Input: part model. Units: mm. Frame: model coordinates. Face numbers are marked on the shaded views. A direction names the side the tool comes from. Round coordinates to 2 decimals unless told otherwise and drop trailing zeros. Loops run counter-clockwise (first coordinate to the right, second up) from the corner with the lowest first, then second, coordinate; pieces in that order, holes last. Notation, with made-up numbers: (13, 80.25) -> (48, 80.25) arc R30 cw to (48, 109.25) -> close; hole circle Ø2 at (11, 43). An arc over 180 degrees is marked (long way). Answer in a Markdown table with one row per item. Add a question column.
Q1. Section C-C, the plane x = 53.5. Output: boundary loops of the cut face in (y, z).
Q2. Section A-A, the plane y = 12.25. Output: boundary loops of the cut face in (x, z).
Q3. Section B-B, the plane x = 0. Output: boundary loops of the cut face in (y, z), and give its area (3 significant figures).
Q4. Reachability of the marked faces 1, 2 and 3 from +Z, -Z, +X, -X, +Y, -Y: full face, straight path, thin tool, end or side. Return the list, or none.
Q5. Pin query (flat end, axial travel): pin 1 (10 mm diameter, centred on x = 30.5, z = -108.5, fed in from -Y); pin 2 (3.5 mm diameter, centred on y = 9, z = -149, fed in from -X); pin 3 (13 mm diameter, centred on y = 15.5, z = -151, fed in from +X); pin 4 (9 mm diameter, centred on x = 0, y = 10, fed in from -Z). Return the tip coordinate at first contact, or that it passes through.
Q6. Section D-D, the plane z = -33.5. Output: boundary loops of the cut face in (x, y).
Q7. Ray query, L1, parallel to X at y = 9, z = -76.5; L2, parallel to X at y = 9.5, z = -77; L3, parallel to X at y = 12, z = -10. Return the intervals inside material, ascending. Write a range as from..to.
```python
from build123d import *

# Parameters (mm, degrees)
BOSS_EXTRUDE1_DEPTH = 2
SKETCH2_W           = 8
SKETCH2_H           = 12
BOSS_EXTRUDE2_DEPTH = 20
SKETCH6_W           = 4
SKETCH6_H           = 2.75
CUT_EXTRUDE3_DEPTH  = 20
SKETCH7_R           = 2
CUT_EXTRUDE4_DEPTH  = 10


with BuildPart() as part:
    # Sketch1 → Boss-Extrude1 (new body)
    with BuildSketch(Plane(origin=(0, 0, 0), x_dir=(1, 0, 0), z_dir=(0, 1, 0))):
        with BuildLine():
            Line((75.074639149, 80.253787975), (10.139177746, 145.189249379))
            ThreePointArc((10.139177746, 145.189249379), (-8.838834765, 161.338834765), (7.310750621, 142.360822254))
            Line((7.310750621, 142.360822254), (71.4177849, 78.253787975))
            Line((71.4177849, 78.253787975), (7.310750621, 14.146753697))
            ThreePointArc((7.310750621, 14.146753697), (-8.838834765, -4.831258814), (10.139177746, 11.318326572))
            Line((10.139177746, 11.318326572), (75.074639149, 76.253787975))
            Line((75.074639149, 76.253787975), (136.907249345, 76.253787975))
            ThreePointArc((136.907249345, 76.253787975), (161.746212025, 78.253787975), (136.907249345, 80.253787975))
            Line((136.907249345, 80.253787975), (75.074639149, 80.253787975))
        make_face()
    extrude(amount=BOSS_EXTRUDE1_DEPTH)

    # Sketch2 → Boss-Extrude2 (add)
    # profile 1 of 3: a face of its own
    with BuildSketch(Plane(origin=(0, 2, 0), x_dir=(1, 0, 0), z_dir=(0, 1, 0))):
        with BuildLine():
            Line((144.496212025, 76.753787975), (144.496212025, 79.503787975))
            ThreePointArc((144.496212025, 79.503787975), (149.346212025, 84.353787975), (154.196212025, 79.503787975))
            Line((154.196212025, 79.503787975), (154.196212025, 76.753787975))
            ThreePointArc((154.196212025, 76.753787975), (149.346212025, 71.903787975), (144.496212025, 76.753787975))
        make_face()
        with BuildLine():
            Line((148.496212025, 76.753787975), (148.496212025, 79.503787975))
            ThreePointArc((148.496212025, 79.503787975), (149.346212025, 80.353787975), (150.196212025, 79.503787975))
            Line((150.196212025, 79.503787975), (150.196212025, 76.753787975))
            ThreePointArc((150.196212025, 76.753787975), (149.346212025, 75.903787975), (148.496212025, 76.753787975))
        make_face(mode=Mode.SUBTRACT)
    # profile 2 of 3: a face of its own
    with BuildSketch(Plane(origin=(0, 2, 0), x_dir=(1, 0, 0), z_dir=(0, 1, 0))):
        with Locations((1.381469518, 5.521849013)):
            Rectangle(SKETCH2_W, SKETCH2_H)
    # profile 3 of 3: a face of its own
    with BuildSketch(Plane(origin=(0, 2, 0), x_dir=(1, 0, 0), z_dir=(0, 1, 0))):
        with Locations((1.381469518, 151.304233441)):
            Rectangle(SKETCH2_W, SKETCH2_H)
    extrude(amount=BOSS_EXTRUDE2_DEPTH)

    # Sketch6 → Cut-Extrude3 (cut)
    with BuildSketch(Plane(origin=(0, 22, 0), x_dir=(1, 0, 0), z_dir=(0, 1, 0))):
        with Locations((152.196212025, 78.128787975)):
            Rectangle(SKETCH6_W, SKETCH6_H)
    extrude(amount=-CUT_EXTRUDE3_DEPTH, mode=Mode.SUBTRACT)

    # Sketch7 → Cut-Extrude4 (cut)
    with BuildSketch(Plane.ZY.offset(2.618530482)):
        with Locations((-5.454118169, 18.296936601)):
            Circle(SKETCH7_R)
        with Locations((-151.053457781, 18.296936601)):
            Circle(SKETCH7_R)
    extrude(amount=-CUT_EXTRUDE4_DEPTH, mode=Mode.SUBTRACT)


solid = part.part
```
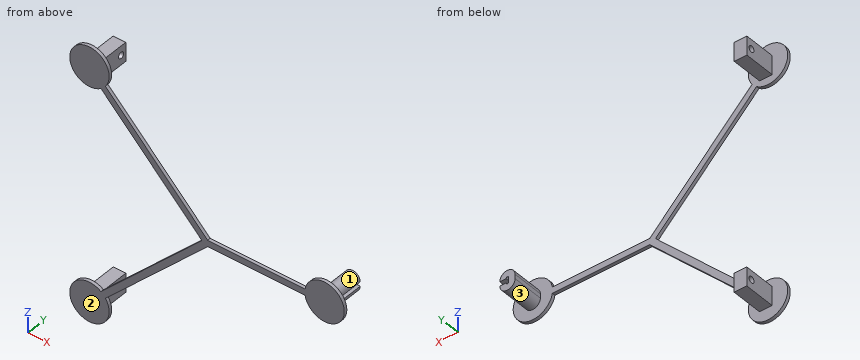
Answer block:
| question | item | result |
|---|---|---|
| 1 | outline | (0, -101.83) -> (2, -101.83) -> (2, -96.17) -> (0, -96.17) -> close; (0, -60.34) -> (2, -60.34) -> (2, -54.68) -> (0, -54.68) -> close |
| 2 | outline | (-2.62, -157.3) -> (5.38, -157.3) -> (5.38, -145.3) -> (-2.62, -145.3) -> close; (-2.62, -11.52) -> (5.38, -11.52) -> (5.38, 0.48) -> (-2.62, 0.48) -> close; (144.5, -79.5) arc R4.85 ccw to (154.2, -79.5) -> (150.2, -79.5) arc R0.85 cw to (148.5, -79.5) -> (148.5, -76.75) arc R0.85 cw to (150.2, -76.75) -> (154.2, -76.75) arc R4.85 ccw to (144.5, -76.75) -> close |
| 3 | outline | (0, -165) -> (2, -165) -> (2, -157.3) -> (22, -157.3) -> (22, -145.3) -> (2, -145.3) -> (2, -140) -> (0, -140) -> close; (0, -16.51) -> (2, -16.51) -> (2, -11.52) -> (22, -11.52) -> (22, 0.48) -> (2, 0.48) -> (2, 8.49) -> (0, 8.49) -> close; hole circle Ø4 at (18.3, -151.05); hole circle Ø4 at (18.3, -5.45) |
| 3 | area | 555 mm^2 |
| 4 | face 1 | +Z, +Y |
| 4 | face 2 | +Z, -Z, +X, -X, -Y |
| 4 | face 3 | -Z, +Y |
| 5 | pin 1 | through |
| 5 | pin 2 | x = -2.62 |
| 5 | pin 3 | x = 5.38 |
| 5 | pin 4 | z = -157.3 |
| 6 | outline | (26.66, 0) -> (32.32, 0) -> (32.32, 2) -> (26.66, 2) -> close |
| 7 | L1 | 144.5..148.53, 150.16..154.19 |
| 7 | L2 | 144.5..148.5 |
| 7 | L3 | -2.62..5.38 |
